Model file for the job. Use its own axes, mm. A direction names the side the tool comes from. Round coordinates to 2 decimals unless told otherwise and drop trailing zeros. Order: outer loops, then holes, each group sorted by start corner. A loop starts at its lowest first (then second) coordinate and runs counter-clockwise, first axis right, second up. Notation, with made-up numbers: (83, 43.5) -> (122, 43.5) arc R18 ccw to (122, 69.5) -> close; hole circle Ø3 at (-14.75, -7). An arc over 180 degrees is marked (long way). Put each result on its own line as item: value. Start each with the question number.
Q1. Probe L1, parallel to X at y = 5, z = 1; L2, parallel to X at y = 2, z = -12.5; L3, parallel to Z at x = 31, y = 3. List the from-to ranges inside material, lowest first.
Q2. Cut at D-D, the plane z = 4.5. List the corners of the cut face in (x, y).
Q3. Cut at B-B, the plane z = -10.5. List the corners of the cut face in (x, y), and give its area (3 significant figures).
Q4. Cut at A-A, the plane x = 7. List the corners of the cut face in (y, z).
Q5. Pull direction Z, two halves, no side cores. Call faces 3 (the face through (-1, 3, 25.4)), 4 (the face through (-18, 3, -12.827)), 5 (the face through (45.244, 3, 0)): released by +Z, released by -Z, zero draft, split by the parting line, or undercut.
Q6. 3-axis set-ups, long thin cutter, end or side, ignore diameter. For faces 1 (the face through (7, 3, -12.827)), 2 (the face through (-1, 0, 0)): which of +Z, -Z, +X, -X, +Y, -Y reach the whole face in a straight line?
Q7. Cut at C-C, the plane y = 2.5. List the corners of the cut face in (x, z).
from build123d import *

# Parameters (mm, degrees)
SKETCH1_W           = 80.9625
SKETCH1_H           = 50.8
BOSS_EXTRUDE1_DEPTH = 6.35
SKETCH3_W           = 6.604
SKETCH3_H           = 25.654
CUT_EXTRUDE1_DEPTH  = 7.35
SKETCH4_W           = 4.7625
SKETCH4_H           = 50.8
BOSS_EXTRUDE2_DEPTH = 6.35
SKETCH5_W           = 12.954
SKETCH5_H           = 19.304
CUT_EXTRUDE2_DEPTH  = 7.35


with BuildPart() as part:
    # Sketch1 → Boss-Extrude1 (new body)
    with BuildSketch(Plane(origin=(0, 0, 0), x_dir=(1, 0, 0), z_dir=(0, 1, 0))):
        Rectangle(SKETCH1_W, SKETCH1_H)
    extrude(amount=BOSS_EXTRUDE1_DEPTH)

    # Sketch3 → Cut-Extrude1 (cut, through all)
    with BuildSketch(Plane(origin=(0, 0, 0), x_dir=(-1, 0, 0), z_dir=(0, -1, 0))):
        with Locations((18.25625, 0)):
            Rectangle(SKETCH3_W, SKETCH3_H)
        with Locations((-7.14375, 0)):
            Rectangle(SKETCH3_W, SKETCH3_H)
    extrude(amount=-CUT_EXTRUDE1_DEPTH, mode=Mode.SUBTRACT)

    # Sketch4 → Boss-Extrude2 (add)
    with BuildSketch(Plane(origin=(0, 6.35, 0), x_dir=(1, 0, 0), z_dir=(0, 1, 0))):
        with Locations((-42.8625, 0)):
            Rectangle(SKETCH4_W, SKETCH4_H)
        with Locations((42.8625, 0)):
            Rectangle(SKETCH4_W, SKETCH4_H)
    extrude(amount=-BOSS_EXTRUDE2_DEPTH)

    # Sketch5 → Cut-Extrude2 (cut, through all)
    with BuildSketch(Plane(origin=(0, 6.35, 0), x_dir=(1, 0, 0), z_dir=(0, 1, 0))):
        with Locations((34.13125, 0)):
            Rectangle(SKETCH5_W, SKETCH5_H)
        with Locations((-34.13125, 0)):
            Rectangle(SKETCH5_W, SKETCH5_H)
    extrude(amount=-CUT_EXTRUDE2_DEPTH, mode=Mode.SUBTRACT)


solid = part.part
Ans:
1. L1: x = -45.24 to -40.61, -27.65 to -21.56, -14.95 to 3.84, 10.45 to 27.65, 40.61 to 45.24
1. L2: x = -45.24 to -21.56, -14.95 to 3.84, 10.45 to 45.24
1. L3: z = -25.4 to -9.65, 9.65 to 25.4
2. outline: (-45.24, 0) -> (-40.61, 0) -> (-40.61, 6.35) -> (-45.24, 6.35) -> close; (-27.65, 0) -> (-21.56, 0) -> (-21.56, 6.35) -> (-27.65, 6.35) -> close; (-14.95, 0) -> (3.84, 0) -> (3.84, 6.35) -> (-14.95, 6.35) -> close; (10.45, 0) -> (27.65, 0) -> (27.65, 6.35) -> (10.45, 6.35) -> close; (40.61, 0) -> (45.24, 0) -> (45.24, 6.35) -> (40.61, 6.35) -> close
3. outline: (-45.24, 0) -> (-21.56, 0) -> (-21.56, 6.35) -> (-45.24, 6.35) -> close; (-14.95, 0) -> (3.84, 0) -> (3.84, 6.35) -> (-14.95, 6.35) -> close; (10.45, 0) -> (45.24, 0) -> (45.24, 6.35) -> (10.45, 6.35) -> close
3. area: 491 mm^2
4. outline: (0, -25.4) -> (6.35, -25.4) -> (6.35, -12.83) -> (0, -12.83) -> close; (0, 12.83) -> (6.35, 12.83) -> (6.35, 25.4) -> (0, 25.4) -> close
5. face 3: released by +Z
5. face 4: undercut
5. face 5: zero draft
6. face 1: +Y, -Y
6. face 2: +Z, -Z, +X, -X, -Y
7. outline: (-45.24, -25.4) -> (45.24, -25.4) -> (45.24, 25.4) -> (-45.24, 25.4) -> close; hole (-40.61, -9.65) -> (-27.65, -9.65) -> (-27.65, 9.65) -> (-40.61, 9.65) -> close; hole (-21.56, -12.83) -> (-14.95, -12.83) -> (-14.95, 12.83) -> (-21.56, 12.83) -> close; hole (3.84, -12.83) -> (10.45, -12.83) -> (10.45, 12.83) -> (3.84, 12.83) -> close; hole (27.65, -9.65) -> (40.61, -9.65) -> (40.61, 9.65) -> (27.65, 9.65) -> close
